from build123d import *

# Parameters (mm, degrees)
SKETCH1_W           = 40.259
SKETCH1_H           = 20.066
BOSS_EXTRUDE1_DEPTH = 38.1
SKETCH2_W           = 54.5
SKETCH2_H           = 18.7198
BOSS_EXTRUDE2_DEPTH = 2.9972
SKETCH3_R           = 2.8702
BOSS_EXTRUDE3_DEPTH = 5.6388
SKETCH4_R           = 1.778
CUT_EXTRUDE1_DEPTH  = 42.513447759
SKETCH5_W           = 7.62
SKETCH5_H           = 2.54
SKETCH5_W_2         = 6.35
CUT_EXTRUDE2_DEPTH  = 42.513447759
FILLET2_R           = 1.27
SKETCH6_W           = 7.239
SKETCH6_H           = 4.318
BOSS_EXTRUDE4_DEPTH = 5.08
BOSS_EXTRUDE4_TAPER = 5
SKETCH7_W           = 4.572
SKETCH7_H           = 20.066
CUT_EXTRUDE3_DEPTH  = 1.524
CHAMFER1_SIZE       = 1.524
CUT_EXTRUDE4_DEPTH  = 1.8542
SKETCH9_R           = 6.75
BOSS_EXTRUDE5_DEPTH = 1.5
CHAMFER2_SIZE       = 0.5
CHAMFER3_SIZE       = 1.5
FILLET3_R           = 0.5
BOSS_EXTRUDE6_DEPTH = 0.5
FILLET4_R           = 1


with BuildPart() as part:
    # Sketch1 → Boss-Extrude1 (new body)
    with BuildSketch(Plane(origin=(0, 0, 0), x_dir=(1, 0, 0), z_dir=(0, 1, 0))):
        Rectangle(SKETCH1_W, SKETCH1_H)
    extrude(amount=BOSS_EXTRUDE1_DEPTH)

    # Sketch2 → Boss-Extrude2 (add)
    with BuildSketch(Plane(origin=(0, 26.67, 0), x_dir=(-1, 0, 0), z_dir=(0, -1, 0))):
        Rectangle(SKETCH2_W, SKETCH2_H)
    extrude(amount=-BOSS_EXTRUDE2_DEPTH)

    # Sketch3 → Boss-Extrude3 (add)
    with BuildSketch(Plane(origin=(0, 38.1, 0), x_dir=(1, 0, 0), z_dir=(0, 1, 0))):
        with Locations(Location((-10.6045, 0, 0), (0, 0, 90))):
            Circle(SKETCH3_R)
    extrude(amount=BOSS_EXTRUDE3_DEPTH)

    # Sketch4 → Cut-Extrude1 (cut, through all)
    with BuildSketch(Plane(origin=(0, 29.6672, 0), x_dir=(1, 0, 0), z_dir=(0, 1, 0))):
        with Locations(Location((-24.5, 5, 0), (0, 0, 270))):
            Circle(SKETCH4_R)
        with Locations(Location((-24.5, -5, 0), (0, 0, 270))):
            Circle(SKETCH4_R)
        with Locations(Location((24.5, -5, 0), (0, 0, 270))):
            Circle(SKETCH4_R)
        with Locations(Location((24.5, 5, 0), (0, 0, 270))):
            Circle(SKETCH4_R)
    extrude(amount=-CUT_EXTRUDE1_DEPTH, mode=Mode.SUBTRACT)

    # Sketch5 → Cut-Extrude2 (cut, through all)
    with BuildSketch(Plane(origin=(0, 29.6672, 0), x_dir=(1, 0, 0), z_dir=(0, 1, 0))):
        with Locations((-28.31, 5)):
            Rectangle(SKETCH5_W, SKETCH5_H)
        with Locations((-27.675, -5)):
            Rectangle(SKETCH5_W_2, SKETCH5_H)
        with Locations((27.675, 5)):
            Rectangle(SKETCH5_W_2, SKETCH5_H)
        with Locations((27.675, -5)):
            Rectangle(SKETCH5_W_2, SKETCH5_H)
    extrude(amount=-CUT_EXTRUDE2_DEPTH, mode=Mode.SUBTRACT)

    # Fillet2
    fillet2_edges = [part.edges().sort_by_distance(p)[0] for p in [
        (27.25, 28.1686, -9.3599),
        (-27.25, 28.1686, 9.3599),
        (27.25, 28.1686, 9.3599),
        (-27.25, 28.1686, -9.3599),
    ]]
    fillet(fillet2_edges, radius=FILLET2_R)

    # Sketch6 → Boss-Extrude4 (add)
    with BuildSketch(Plane.ZY.offset(20.1295)):
        with Locations((0, 5.715)):
            Rectangle(SKETCH6_W, SKETCH6_H)
    extrude(amount=BOSS_EXTRUDE4_DEPTH, taper=BOSS_EXTRUDE4_TAPER)

    # Sketch7 → Cut-Extrude3 (cut)
    with BuildSketch(Plane(origin=(0, 38.1, 0), x_dir=(1, 0, 0), z_dir=(0, 1, 0))):
        with Locations((17.8435, 0)):
            Rectangle(SKETCH7_W, SKETCH7_H)
    extrude(amount=-CUT_EXTRUDE3_DEPTH, mode=Mode.SUBTRACT)

    # Chamfer1
    chamfer1_edges = [part.edges().sort_by_distance(p)[0] for p in [
        (15.5575, 38.1, 0),
    ]]
    chamfer(chamfer1_edges, length=CHAMFER1_SIZE - 0.0001)  # a hair under: the kernel refuses the full size

    # Sketch8 → Cut-Extrude4 (cut)
    with BuildSketch(Plane(origin=(0, 38.1, 0), x_dir=(1, 0, 0), z_dir=(0, 1, 0))):
        with BuildLine():
            Line((-10.6045, 10.121534413), (-31.431367674, 17.812165279))
            Line((-31.431367674, 17.812165279), (-23.526690426, -15.868179363))
            Line((-23.526690426, -15.868179363), (-10.6045, -10.033))
            ThreePointArc((-10.6045, -10.033), (-20.1295, 0.044267206), (-10.6045, 10.121534413))
        make_face()
    extrude(amount=-CUT_EXTRUDE4_DEPTH, mode=Mode.SUBTRACT)

    # Sketch9 → Boss-Extrude5 (add)
    with BuildSketch(Plane(origin=(0, 38.1, 0), x_dir=(1, 0, 0), z_dir=(0, 1, 0))):
        with Locations(Location((-10.6045, 0, 0), (0, 0, 90))):
            Circle(SKETCH9_R)
    extrude(amount=BOSS_EXTRUDE5_DEPTH)

    # Chamfer2
    chamfer2_edges = [part.edges().sort_by_distance(p)[0] for p in [
        (1.274211255, 38.1, -10.033),
    ]]
    chamfer(chamfer2_edges, length=CHAMFER2_SIZE)
    chamfer2_2_edges = [part.edges().sort_by_distance(p)[0] for p in [
        (-20.022463004, 38.1, 1.421765307),
    ]]
    chamfer(chamfer2_2_edges, length=CHAMFER2_SIZE)
    chamfer2_3_edges = [part.edges().sort_by_distance(p)[0] for p in [
        (-10.6045, 39.6, 6.75),
    ]]
    chamfer(chamfer2_3_edges, length=CHAMFER2_SIZE)

    # Chamfer3
    chamfer3_edges = [part.edges().sort_by_distance(p)[0] for p in [
        (0, 0, 10.033),
        (-20.1295, 0, 0),
        (0, 0, -10.033),
        (20.1295, 0, 0),
    ]]
    chamfer(chamfer3_edges, length=CHAMFER3_SIZE)

    # Fillet3
    fillet3_edges = [part.edges().sort_by_distance(p)[0] for p in [
        (20.1295, 19.038, 10.033),
        (20.1295, 19.038, -10.033),
        (-20.1295, 18.8729, 10.033),
        (-20.1295, 18.8729, -10.033),
    ]]
    fillet(fillet3_edges, radius=FILLET3_R)

    # Sketch12 → Boss-Extrude6 (add, symmetric)
    with BuildSketch(Plane.XY):
        Polygon((-27.25, 29.6672), (-20.1295, 29.6672), (-20.1295, 30.6672), align=None)
    boss_extrude6 = extrude(amount=BOSS_EXTRUDE6_DEPTH, both=True)

    # Mirror1: Boss-Extrude6 across plane
    add(boss_extrude6.mirror(Plane(origin=(0, 0, 0), x_dir=(0, 0, 1), z_dir=(1, 0, 0))))

    # Fillet4
    fillet4_edges = [part.edges().sort_by_distance(p)[0] for p in [
        (-22.6695, 3.778221205, 3.397278795),
        (-22.6695, 7.651778795, 3.397278795),
        (-22.6695, 7.651778795, -3.397278795),
        (-22.6695, 3.778221205, -3.397278795),
        (-25.2095, 5.715, 3.175057589),
        (-25.2095, 7.429557589, 0),
        (-25.2095, 5.715, -3.175057589),
        (-25.2095, 4.000442411, 0),
    ]]
    fillet(fillet4_edges, radius=FILLET4_R)


solid = part.part
Part model, mm, in its own coordinate system. A direction names the side the tool comes from. Coordinates: 2 decimals unless noted, no trailing zeros. Write each loop counter-clockwise with the first axis right and the second up, starting at its lowest first coordinate (ties: lowest second). Pieces come first, ordered by that corner, then holes. Notation, with made-up numbers: M -34,57.25 L -6,57.25 A15 ccw -6,66.25 Z; hole C 73.5,32.5 d2. An arc over 180 degrees is marked long. Return JSON: item names as keys, results as strings.
1. Saw through at C-C, the plane x = 17. Write the cut outline in (y, z), then the cut area to 3 significant figures.
Determined:
{"outline": "M 0,-8.53 L 1.5,-10.03 L 36.58,-10.03 L 36.58,10.03 L 1.5,10.03 L 0,8.53 Z", "area": "732 mm²"}
2. Probe L1, parallel to Z at x = -24.5, y = 27.5; L2, parallel to Y at x = 9.5, z = 1.75; L3, parallel to X at y = 27.45, z = 5. List the from-to ranges inside material, lowest first.
Determined:
{"L1": "-9.36 to -6.78, -3.22 to 3.22, 6.78 to 9.36", "L2": "0 to 38.1", "L3": "-22.72 to 22.72"}
3. 3-axis set-ups, long thin cutter, end or side, ignore diameter. For faces 1 (the face through (23, 28, 9.36)), 2 (the face through (23, 26.67, 0)), 3 (the face through (26, 28, 6.27)), 4 (the face through (22, 29.667, -5)): which of +Z, -Z, +X, -X, +Y, -Y reach the whole face in a straight line?
Determined:
{"face 1": "+Z, +X, +Y, -Y", "face 2": "+Z, -Z, +X, -Y", "face 3": "+X, +Y, -Y", "face 4": "-Z, +X, +Y"}
4. Flat gauge pins, fed straight in: pin 1 Ø5 at (x, z) = (-17, 5.5) entering from +Y; pin 2 Ø0.8 at (x, y) = (26.5, 28) entering from -Z; pin 3 Ø0.5 at (x, y) = (-22.5, 30) entering from +Z; pin 4 Ø0.8 at (x, y) = (24.5, 30.5) entering from +Z. Where does each tip first touch, or does it go through?
Determined:
{"pin 1": "y = 39.6", "pin 2": "z = -9.35", "pin 3": "z = 0.5", "pin 4": "through"}
5. Pull direction Y, two halves, no side cores. Call faces 5 (the face through (-23, 26.67, 0)), 6 (the face through (-18, 36.246, 8)), 7 (the face through (-23, 28, -9.36)): pulls with the +Y half, pulls with the -Y half, needs draft (parallel to the pull), parting line crosses it, or undercut.
Determined:
{"face 5": "undercut", "face 6": "pulls with the +Y half", "face 7": "needs draft"}
6. Saw through at A-A, the plane x = 24.5. Write the cut outline in (y, z).
Determined:
{"outline": "M 26.67,-9.36 L 29.67,-9.36 L 29.67,-6.78 L 26.67,-6.78 Z; M 26.67,-3.22 L 29.67,-3.22 L 29.67,-0.5 L 30.05,-0.5 L 30.05,0.5 L 29.67,0.5 L 29.67,3.22 L 26.67,3.22 Z; M 26.67,6.78 L 29.67,6.78 L 29.67,9.36 L 26.67,9.36 Z"}
7. Saw through at B-B, the plane y = 34.5. Write the cut outline in (x, z).
Determined:
{"outline": "M -20.13,-9.53 A0.5 ccw -19.63,-10.03 L 19.63,-10.03 A0.5 ccw 20.13,-9.53 L 20.13,9.53 A0.5 ccw 19.63,10.03 L -19.63,10.03 A0.5 ccw -20.13,9.53 Z"}
